Autodesk Fusion 360 part; units mm, degrees
sketch "Sketch1" plane through (0, 0, 0) normal (0, 0, 1) x (1, 0, 0)
  circle A0 centre (0, 0) radius 25
  dimension "d1" = 50
extrude "Extrude1" add sketch "Sketch1" along normal blind 2.5
sketch "Sketch2" plane through (0, 0, 2.5) normal (0, 0, 1) x (-1, 0, 0)
  circle A0 centre (0, 0) radius 25
  circle A1 centre (0, 0) radius 23
  circle A2 centre (0, 0) radius 21 construction
  circle A3 centre (0, 0) radius 4
  line L0 (0, 0) -> (0, -21) construction
  line L1 (0, 0) -> (-18.1865, 10.5) construction
  line L2 (18.1865, 10.5) -> (0, 0) construction
  line L3 (18.1865, 10.5) -> (0, -21) construction
  line L4 (-18.1865, 10.5) -> (0, -21) construction
  line L5 (-18.1865, 10.5) -> (18.1865, 10.5) construction
  circle A4 centre (0, 0) radius 5
  circle A5 centre (0, 0) radius 15 construction
  circle A6 centre (0, -15) radius 6
  circle A7 centre (-12.9904, 7.5) radius 6
  circle A8 centre (12.9904, 7.5) radius 6
  line L6 (8.5332, 3.4833) -> (3.9156, 0.8173)
  line L7 (7.2832, 5.6484) -> (2.6656, 2.9824)
  line L8 (8.5332, 3.4833) -> (7.2832, 5.6484) construction
  line L9 (3.9156, 0.8173) -> (2.6656, 2.9824) construction
  line L10 (-7.2832, 5.6484) -> (-2.6656, 2.9824)
  line L11 (-8.5332, 3.4833) -> (-3.9156, 0.8173)
  line L12 (-2.6656, 2.9824) -> (-3.9156, 0.8173) construction
  line L13 (-7.2832, 5.6484) -> (-8.5332, 3.4833) construction
  line L14 (-1.25, -9.1317) -> (-1.25, -3.7997)
  line L15 (1.25, -9.1317) -> (1.25, -3.7997)
  line L16 (-1.25, -3.7997) -> (1.25, -3.7997) construction
  line L17 (-1.25, -9.1317) -> (1.25, -9.1317) construction
  circle A9 centre (0, 0) radius 7.5
  line L18 (5.071, 5.5258) -> (2.7419, 4.1811)
  line L19 (7.321, 1.6287) -> (4.9919, 0.284)
  line L20 (-7.321, 1.6287) -> (-4.9919, 0.284)
  line L21 (-5.071, 5.5258) -> (-2.7419, 4.1811)
  line L22 (2.25, -7.1545) -> (2.25, -4.4651)
  line L23 (-2.25, -7.1545) -> (-2.25, -4.4651)
  dimension "d4" = -2
  dimension "d5" = -4
  dimension "d6" = 8
  dimension "d7" = 1
  dimension "d8" = -10
  dimension "d13" = 360
  dimension "d14" = 2.5
  dimension "d15" = 3.5
  dimension "d17" = 360
  dimension "d20" = 1
extrude "Extrude2" add sketch "Sketch2" along normal blind 1.5 contours A0 | A3 | A4 L6 L7 A9 | A4 L14 L15 A9 | A4 A9 L19 L22 | A8 L6 L7 A9 | A6 L14 L15 A9 | A4 L10 L11 A9 | A4 A9 L18 L21 | A8 | A4 A9 L20 L23 | A6 | A7 L10 L11 A9 | A7
Geometry: final body of the model. Coordinates: model frame, mm. A direction names the side the tool comes from. Give positions to 0.01 mm unless a question says otherwise; leave off trailing zeros. Write each loop counter-clockwise with the first axis right and the second up, starting at its lowest first coordinate (ties: lowest second). Pieces come first, ordered by that corner, then holes.
(1) First-contact query: P1, Ø4, axis at x = 7, y = -10.5, coming from the -Z side; P2, Ø0.8, axis at y = 6.5, z = 3.5, coming from the -X side; P3, Ø1.6, axis at y = 7.5, z = 3.5, coming from the -X side; P4, Ø3, axis at x = -10, y = 2.5, coming from the +Z side. Flat tips, straight axial feed; report the tip coordinate or a pass-through.
(2) Access query for faces 3 (the flat face through (0, 0, 4)), 4 (the flat face through (-6.701, -2.426, 3.24)). Directions: +Z, -Z, +X, -X, +Y, -Y. A direction counts if a zero-diameter tool reaches every point of the face in a straight line with its end or side. Return the directions, or none.
(3) Ray query, line 1 (X direction, y = 8, z = 3.25); line 2 (Y direction, x = 11, z = 2.75); line 3 (Z direction, x = -15, y = 5). Return the intervals inside material, ascending.
(4) Mould query, pull axis Y, two halves, no side actions, for faces 1 (the cylindrical face through (4, 3, 3)), 2 (the flat face through (0, 15, 4)). Classes: released by +Y, released by -Y, zero draft, split by the parting line, or undercut.
(5) Cut plane A-A, the plane z = 1.5. Return loops of the section in (x, y), then the cut area to 3 significant figures.
Values follow:
1. P1: stops at z = 0
1. P2: stops at x = -24.24
1. P3: stops at x = -24.09
1. P4: stops at z = 2.5
2. face 3: +Z, +X, -X, +Y, -Y
2. face 4: +Z
3. line 1: x = -23.69 to -21.56, -1.25 to 1.25, 21.56 to 23.69
3. line 2: y = -22.45 to -20.2, -13.16 to -1.84, 20.2 to 22.45
3. line 3: z = 0 to 2.5
4. face 1: undercut
4. face 2: zero draft
5. outline: circle Ø50 at (0, 0)
5. area: 1,960 mm2
